Geometry check sheet. Reference: drawing and pictorial views, mm from the part's lowest x, y, z. A direction names the side the tool comes from. Coordinates: 2 decimals unless noted, no trailing zeros. Loops run counter-clockwise (first coordinate to the right, second up) from the corner with the lowest first, then second, coordinate; pieces in that order, holes last.
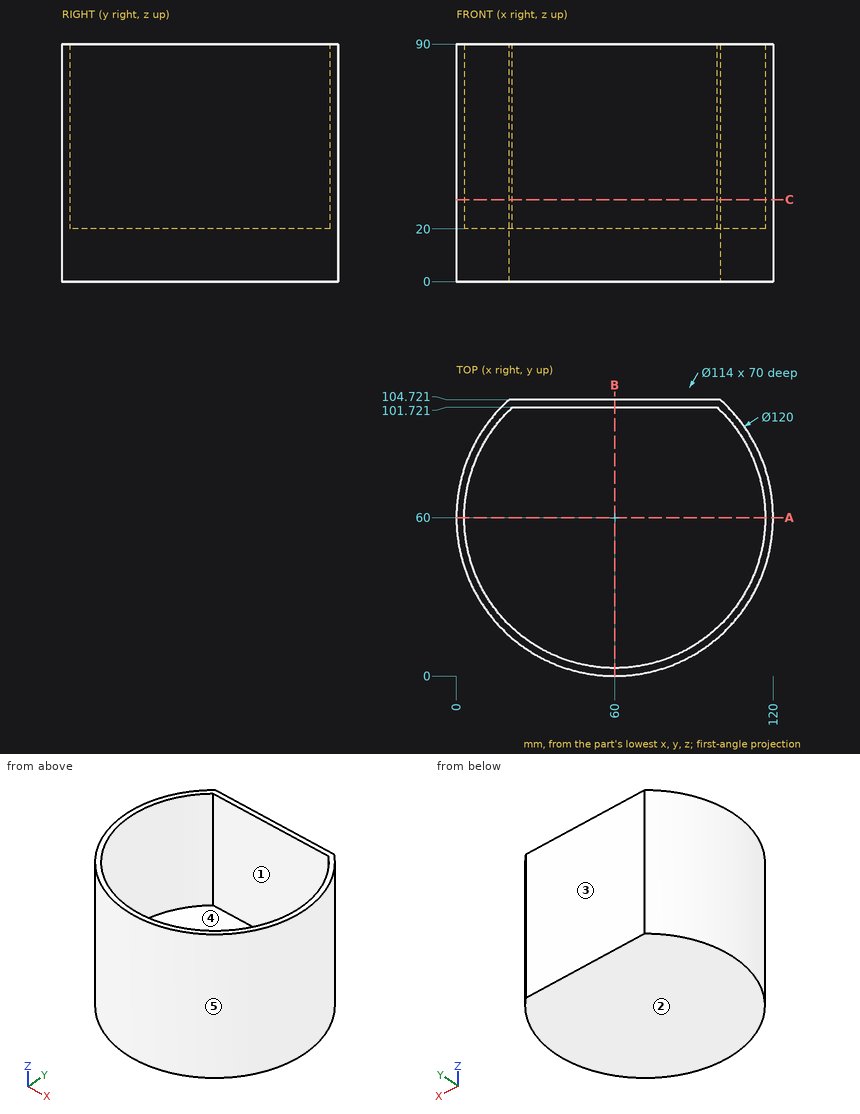
1) Material ranges on probe 1 along X at (y, z) = (60, 47); probe 2 along Z at (x, y) = (57, 63.5); probe 3 along X at (y, z) = (37.5, 41.5), recorded low to high.
Data:
probe 1: x = 0 to 3, 117 to 120
probe 2: z = 0 to 20
probe 3: x = 4.38 to 7.63, 112.37 to 115.62
2) Mould release check, pull along X, two halves, no side actions. Record for the marked faces 3, 4 and 5: +X half, -X half, draft (parallel to the pull), parting line (faces both ways), or undercut.
Data:
face 3: draft
face 4: undercut
face 5: parting line
3) Section check B-B on x = 60. Record the cut outline in (y, z).
Data:
outline: (0, 0) - (104.72, 0) - (104.72, 90) - (101.72, 90) - (101.72, 20) - (3, 20) - (3, 90) - (0, 90) - close
4) Section check C-C on z = 31. Record the cut outline in (x, y).
Data:
outline: (20, 104.72) arc R60 ccw (long way) to (100, 104.72) - close; hole (21.16, 101.72) arc R57 ccw (long way) to (98.84, 101.72) - close
5) Depth check by flat-ended pin: pin 1 (8 mm diameter, centred on x = 90.5, y = 58.5, fed in from +Z); pin 2 (8 mm diameter, centred on x = 41.5, y = 13, fed in from -Z); pin 3 (12 mm diameter, centred on y = 39, z = 55.5, fed in from +X) (1 decimal); pin 4 (2 mm diameter, centred on y = 51.5, z = 67, fed in from +X). Enter the tip coordinate at first touch or a pass-through.
Data:
pin 1: stops at z = 20
pin 2: stops at z = 0
pin 3: stops at x = 118.1
pin 4: stops at x = 119.53
6) Section check A-A on y = 60. Record the cut outline in (x, z), and give its area (3 significant figures).
Data:
outline: (0, 0) - (120, 0) - (120, 90) - (117, 90) - (117, 20) - (3, 20) - (3, 90) - (0, 90) - close
area: 2,820 mm2
7) Access from +Z, -Z, +X, -X, +Y, -Y to the whole of each face (thin tool, end or side, straight path). Record for the marked faces 1 and 2.
Data:
face 1: +Z
face 2: -Z, +X, -X, +Y, -Y
